The drawing under review shows one solid part. Ordinate dimensions are in mm from its lowest x, y, z. A direction names the side the tool comes from. Round coordinates to 2 decimals unless told otherwise and drop trailing zeros. Write each loop counter-clockwise with the first axis right and the second up, starting at its lowest first coordinate (ties: lowest second). Pieces come first, ordered by that corner, then holes.
Item 1: Clearance check with flat-ended pins moving along their axes: pin 1 Ø1.7 at (x, z) = (14.5, 1.5) entering from +Y; pin 2 Ø3 at (x, y) = (2.5, 15.75) entering from +Z; pin 3 Ø1.7 at (x, z) = (14.5, 6) entering from +Y (1 decimal). State where each tip first meets the part, or that it passes through.
Item 2: Machinability: for the marked faces 1, 2, 3, 4 and 5, which of the approach directions +Z, -Z, +X, -X, +Y, -Y give a long, thin tool a straight path to every point of the face, cutting with its end or side? Answer none if there is none.
Item 3: Add section A-A (z = 2.25). Give the boundary of the cut face in (x, y).
Item 4: Add section D-D (z = 4.25). Give the boundary of the cut face in (x, y).
Item 5: Add section B-B (y = 7.5). Give the boundary of the cut face in (x, z) (1 decimal).
Item 6: To check wall thickness, follow L1, parallel to Y at x = 12.5, z = 7.5 (1 decimal); L2, parallel to Y at x = 20, z = 0.5; L3, parallel to Z at x = 19.5, y = 21. State the ranges of each line that lie inside material, in increasing order.
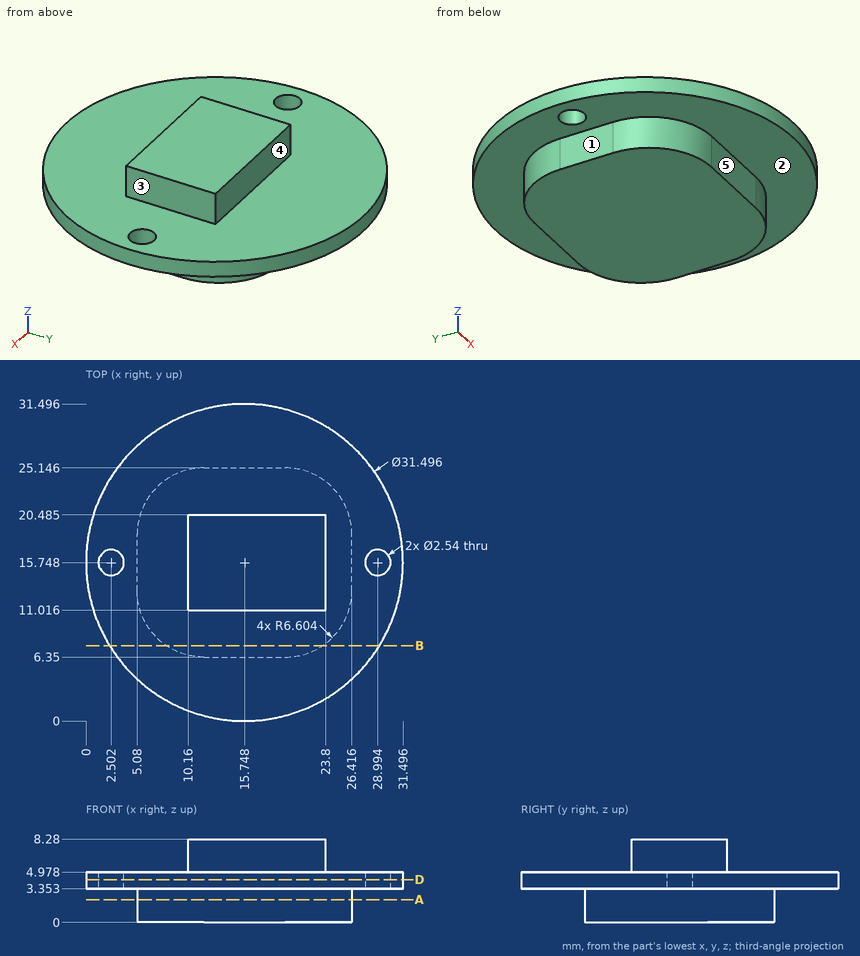
Numbers:
1. pin 1: stops at y = 25.15
1. pin 2: stops at z = 4.98
1. pin 3: stops at y = 20.5
2. face 1: -Z, -X, +Y, -Y
2. face 2: -Z
2. face 3: +Z, +X, +Y, -Y
2. face 4: +Z, +X, -X, +Y
2. face 5: -Z, +X, -X, -Y
3. outline: (5.08, 12.95) arc R6.6 ccw to (11.68, 6.35) - (19.81, 6.35) arc R6.6 ccw to (26.42, 12.95) - (26.42, 18.54) arc R6.6 ccw to (19.81, 25.15) - (11.68, 25.15) arc R6.6 ccw to (5.08, 18.54) - close
4. outline: circle Ø31.5 at (15.75, 15.75); hole circle Ø2.54 at (2.5, 15.75); hole circle Ø2.54 at (28.99, 15.75)
5. outline: (2.3, 3.4) - (8, 3.4) - (8, 0) - (23.5, 0) - (23.5, 3.4) - (29.2, 3.4) - (29.2, 5) - (2.3, 5) - close
6. L1: y = 11 to 20.5
6. L2: y = 6.35 to 25.14
6. L3: z = 0 to 4.98
